Here's the drawing with two shaded views (mm, measured from the low corner). I have some questions. A direction names the side the tool comes from. Coordinates: 2 decimals unless noted, no trailing zeros. Write each loop counter-clockwise with the first axis right and the second up, starting at its lowest first coordinate (ties: lowest second). Pieces come first, ordered by that corner, then holes. Notation, with made-up numbers: (-6, 78) - (4, 78) arc R18 ccw to (4, 109) - close; hole circle Ø7 at (-36.5, 40). An arc over 180 degrees is marked (long way). Answer in a Markdown table with one row per item. Add a question column.
Item 1: Which directions (+Z, -Z, +X, -X, +Y, -Y) give clear straight access to the entire face, cutting with the end or side of a thin tool? Please do the marked faces 5, 6 and 7.
Item 2: We'd pull the mould along Y, two halves only. Please class the marked faces 1, 2, 3 and 4: +Y half, -Y half, draft (parallel to the pull), parting line (faces both ways), or undercut.
Item 3: I'm going to push flat-ended pins straight in: pin 1 (23 mm diameter, centred on y = 83, z = 79, fed in from +X); pin 2 (3 mm diameter, centred on x = 64, y = 53, fed in from +Z); pin 3 (15.5 mm diameter, centred on x = 34, y = 76.5, fed in from +Z). Where does each tip first touch, or does it pass through?
Item 4: Imagine slicing it at A-A (z = 109.5). Please give me the cut outline in (x, y), plus the area to 3 significant figures.
Item 5: Imagine slicing it at D-D (y = 88). Please give me the cut outline in (x, z), plus the area to 3 significant figures.
Item 6: Imagine slicing it at B-B (x = 125). Please give me the cut outline in (y, z), plus the area to 3 significant figures.
Item 7: Imagine slicing it at C-C (x = 15.5). Please give me the cut outline in (y, z).
Item 8: If I drill on probe 1 along Y at (x, z) = (148.5, 21); probe 2 along Z at (x, y) = (61, 38.5); probe 3 along X at (y, z) = (6, 101), over which ranges is the centre line in solid material (lowest first)? Write a range as from..to.
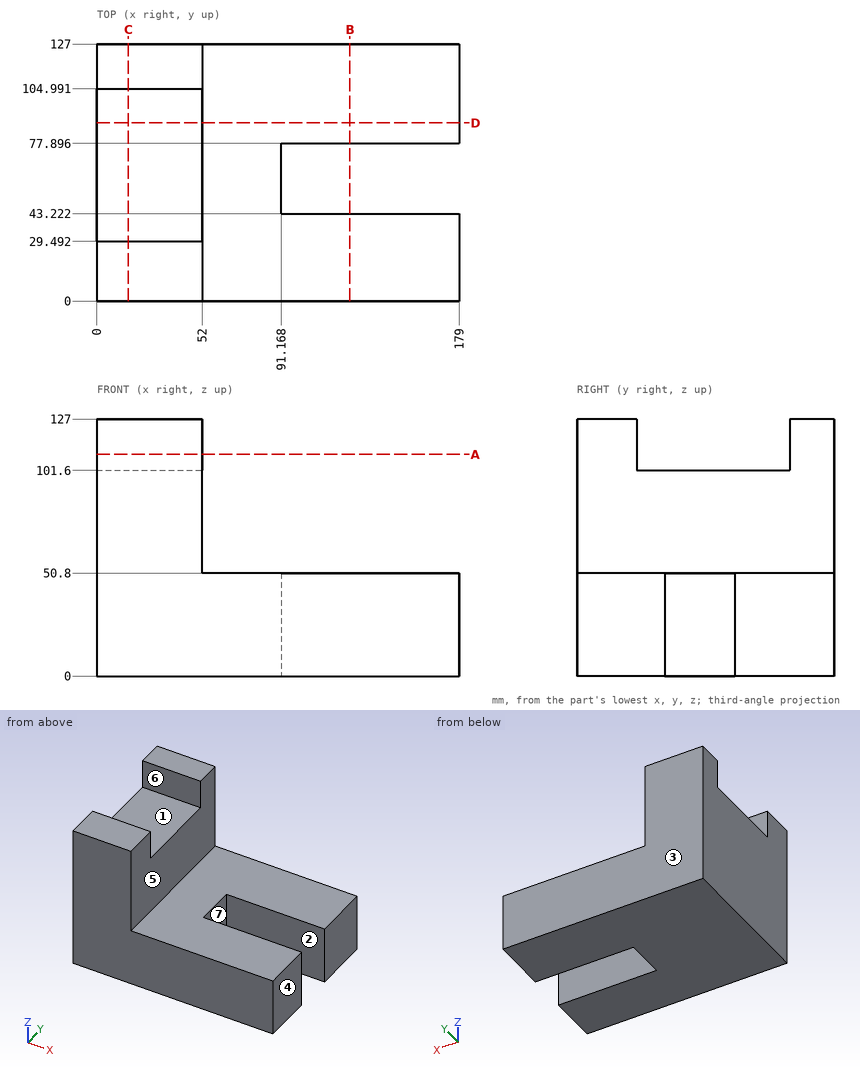
Here are the results:
| question | item | result |
|---|---|---|
| 1 | face 5 | +Z, +X, +Y, -Y |
| 1 | face 6 | +Z, +X, -X |
| 1 | face 7 | +Z, -Z, +X |
| 2 | face 1 | undercut |
| 2 | face 2 | undercut |
| 2 | face 3 | +Y half |
| 2 | face 4 | draft |
| 3 | pin 1 | stops at x = 52 |
| 3 | pin 2 | stops at z = 50.8 |
| 3 | pin 3 | stops at z = 101.6 |
| 4 | outline | (0, 0) - (52, 0) - (52, 29.49) - (0, 29.49) - close; (0, 104.99) - (52, 104.99) - (52, 127) - (0, 127) - close |
| 4 | area | 2,680 mm2 |
| 5 | outline | (0, 0) - (179, 0) - (179, 50.8) - (52, 50.8) - (52, 101.6) - (0, 101.6) - close |
| 5 | area | 11,700 mm2 |
| 6 | outline | (0, 0) - (43.22, 0) - (43.22, 50.8) - (0, 50.8) - close; (77.9, 0) - (127, 0) - (127, 50.8) - (77.9, 50.8) - close |
| 6 | area | 4,690 mm2 |
| 7 | outline | (0, 0) - (127, 0) - (127, 127) - (104.99, 127) - (104.99, 101.6) - (29.49, 101.6) - (29.49, 127) - (0, 127) - close |
| 8 | probe 1 | y = 0..43.22, 77.9..127 |
| 8 | probe 2 | z = 0..50.8 |
| 8 | probe 3 | x = 0..52 |
